Autodesk Inventor part; units mm, degrees
ref_plane "YZ Plane" through (0, 0, 0) normal (1, 0, 0) x (0, 1, 0)
ref_plane "XZ Plane" through (0, 0, 0) normal (0, 1, 0) x (-1, 0, 0)
ref_plane "XY Plane" through (0, 0, 0) normal (0, 0, 1) x (1, 0, 0)
sketch "Sketch1" plane through (0, 0, 0) normal (0, 0, 1) x (1, 0, 0)
  line L0 (0, 0) -> (0, 39)
  line L1 (42, 0) -> (42, 25.5)
  line L2 (42, 25.5) -> (36, 25.5)
  line L3 (36, 25.5) -> (36, 23)
  line L4 (36, 23) -> (25, 23)
  line L5 (25, 23) -> (25, 27)
  line L6 (25, 27) -> (26.7321, 30)
  line L7 (26.7321, 30) -> (42.5, 30)
  line L8 (42.5, 30) -> (42.5, 39)
  line L9 (42.5, 39) -> (52, 39)
  line L10 (52, 39) -> (52, 11)
  line L11 (52, 11) -> (100, 11)
  line L12 (100, 11) -> (100, 0)
  line L13 (100, 0) -> (42, 0)
  dimension "d0" = 39
  dimension "d1" = 200
  dimension "d2" = 84
  dimension "d3" = 85
  dimension "d4" = 11
  dimension "d5" = 50
  dimension "d6" = 72
  dimension "d7" = 23
  dimension "d8" = 30
  dimension "d9" = 30
  dimension "d10" = 25.5
  dimension "d11" = 104
  dimension "d12" = 3
revolve "Revolution1" add sketch "Sketch1" angle 360 about axis through (0, 0, 0) along (0, 1, 0)
sketch "Sketch2" plane through (0, 0, 0) normal (1, 0, 0) x (0, 1, 0)
  line L0 (18, 23) -> (12, 23)
  line L1 (12, 23) -> (12, 7)
  line L2 (12, 7) -> (18, 7)
  line L3 (18, 7) -> (18, 23)
  line L4 (0, -42) -> (0, 42)
  point P0 (0, 0)
  point P1 (0, 0)
  dimension "d14" = 12
  dimension "d15" = 6
  dimension "d16" = 16
  dimension "d17" = 7
extrude "Extrusion1" cut sketch "Sketch2" along normal through all both and the other way through all
mirror "Mirror1" about plane through (0, 0, 0) normal (0, 0, 1) of "Extrusion1"
sketch "Sketch3" plane through (0, 11, 0) normal (0, 1, 0) x (1, 0, 0)
  circle A0 centre (0, 0) radius 52
  circle A1 centre (0, 0) radius 100
  line L0 (99.6795, 8) -> (80, 8)
  arc A2 (80, 8) -> (80, -8) centre (80, 0) ccw
  line L1 (80, -8) -> (99.6795, -8)
  arc A3 (99.6795, -8) -> (99.6795, 8) centre (0, 0) ccw
  dimension "d20" = 8
  dimension "d21" = 80
extrude "Extrusion2" cut sketch "Sketch3" against normal through all contours A1 L1 A2 L0 picked at (86.6667, 0)
sketch "Sketch4" plane through (80, 11, -8) normal (0, 1, 0) x (1, 0, 0)
  circle A0 centre (-80, -8) radius 52
  line L0 (-80, -8) -> (-34.0381, 37.9619) construction
  line L1 (-80, -8) -> (-15, -8) construction
  line L2 (-54.4876, 37.3114) -> (-43.9376, 47.8614)
  arc A1 (-24.1386, 28.0624) -> (-43.9376, 47.8614) centre (-34.0381, 37.9619) ccw
  line L3 (-24.1386, 28.0624) -> (-34.6886, 17.5124)
  dimension "d24" = 65
  dimension "d25" = 45
  dimension "d26" = 14
extrude "Extrusion3" add sketch "Sketch4" along normal blind 24 contours A0 L2 A1 L3
sketch "Sketch5" plane through (80, 35, -8) normal (0, 1, 0) x (1, 0, 0)
  arc A0 (-24.1386, 28.0624) -> (-43.9376, 47.8614) centre (-34.0381, 37.9619) ccw
  point P0 (-80, -8)
hole "Hole1" at (45.9619, 35, -45.9619) direction (0, -1, 0) diameter 12 end through all
pattern_circular "Circular Pattern1" count 4 over 360 about axis through (0, 5.5, 0) along (0, 1, 0) of "Extrusion2", "Extrusion3", "Hole1"
properties part number "Part038. Flat stand" material "Steel, Carbon"
The model under review builds one solid part; all positions refer to its coordinate system, in mm. A direction names the side the tool comes from. Give positions to 0.01 mm unless a question says otherwise; leave off trailing zeros. Write each loop counter-clockwise with the first axis right and the second up, starting at its lowest first coordinate (ties: lowest second). Pieces come first, ordered by that corner, then holes. Notation, with made-up numbers: M -30.75,-13.5 L -8.75,-13.5 A18 ccw -8.75,8.5 Z; hole C 47,41.25 d1. An arc over 180 degrees is marked long. One line per question, with ' | ' between items. Start each with the question number.
Item 1: We need section A-A on z = 0. Write out the cut boundary in (x, y).
Item 2: For pin 1 (4 mm diameter, centred on y = 22, z = -45.5, fed in from -X); pin 2 (12 mm diameter, centred on x = -72.5, y = 19, fed in from +Z); pin 3 (1.8 mm diameter, centred on x = 41, y = 15, fed in from +Z); pin 4 (10 mm diameter, centred on x = 1, z = 70.5, fed in from +Y), all flat-tipped, find the tip position at first contact; note any pin that passes through.
Item 3: For faces 4 (the flat face through (43, 18, -15)), 5 (the flat face through (-50.5, 22.8, -30.7)), 6 (the flat face through (46, 35, -39)), 7 (the cylindrical face through (-33.727, 34.563, 25.861)), list the 3-axis set-ups (+Z, -Z, +X, -X, +Y, -Y) from which the entire face can be reached by the end or side of a thin tool; tool diameter is ignored.
Item 4: Draft analysis for pull direction Z (two halves, no side actions). For faces 1 (the flat face through (-30.9, 22.8, -50.7)), 2 (the flat face through (90, 6, 8)), 3 (the flat face through (-39, 35, -46)), state which applies: released by +Z, released by -Z, zero draft, split by the parting line, or undercut.
Item 5: We need section B-B on x = 0. Write out the cut boundary in (y, z).
Item 6: Wall thickness on line 1 (X direction, y = 32, z = 0); line 2 (X direction, y = 21.5, z = 44.5); line 3 (X direction, y = 19.5, z = -45): over which ranges is each line inside the solid? List them lowest first. Write a range as from..to.
Item 7: We need section D-D on z = -77.5. Write out the cut boundary in (x, y), plus the area to 3 significant figures.
Item 8: We need section C-C on y = 8. Write out the cut boundary in (x, z), plus the area to 3 significant figures.
Results found:
1) outline: M -72,0 L -42,0 L -42,25.5 L -36,25.5 L -36,23 L -25,23 L -25,27 L -26.73,30 L -42.5,30 L -42.5,39 L -52,39 L -52,11 L -72,11 Z; M 25,23 L 36,23 L 36,25.5 L 42,25.5 L 42,0 L 72,0 L 72,11 L 52,11 L 52,39 L 42.5,39 L 42.5,30 L 26.73,30 L 25,27 Z
2) pin 1: stops at x = -59.96 | pin 2: passes through | pin 3: stops at z = 59.36 | pin 4: stops at y = 11
3) face 4: +X, -X | face 5: -X, +Y | face 6: -Z, +X, +Y | face 7: +Y
4) face 1: released by -Z | face 2: undercut | face 3: zero draft
5) outline: M 0,-72 L 11,-72 L 11,-52 L 39,-52 L 39,-42.5 L 30,-42.5 L 30,-26.73 L 27,-25 L 23,-25 L 23,-36 L 25.5,-36 L 25.5,-42 L 0,-42 Z; M 0,42 L 25.5,42 L 25.5,36 L 23,36 L 23,25 L 27,25 L 30,26.73 L 30,42.5 L 39,42.5 L 39,52 L 11,52 L 11,72 L 0,72 Z
6) line 1: x = -52..-42.5, 42.5..52 | line 2: x = -59.89..-51.78, -40.14..40.14, 51.78..59.89 | line 3: x = -59.93..-51.88, -40.04..40.04, 51.88..59.93
7) outline: M -63.2,0 L -7.6,0 L -7.6,11 L -63.2,11 Z; M 7.6,0 L 63.2,0 L 63.2,11 L 7.6,11 Z | area: 1,220 mm2
8) outline: M -99.68,-8 A100 ccw -8,-99.68 L -8,-80 A8 cw 8,-80 L 8,-99.68 A100 ccw 99.68,-8 L 80,-8 A8 cw 80,8 L 99.68,8 A100 ccw 8,99.68 L 8,80 A8 cw -8,80 L -8,99.68 A100 ccw -99.68,8 L -80,8 A8 cw -80,-8 Z; hole C -45.96,-45.96 d12; hole C -45.96,45.96 d12; hole C 0,0 d84; hole C 45.96,-45.96 d12; hole C 45.96,45.96 d12 | area: 23,700 mm2
